Geometry check sheet. Reference: the model listing, model coordinates, mm. A direction names the side the tool comes from. Round coordinates to 2 decimals unless told otherwise and drop trailing zeros. Loops run counter-clockwise (first coordinate to the right, second up) from the corner with the lowest first, then second, coordinate; pieces in that order, holes last. Notation, with made-up numbers: M 49,50 L 94,50 A23 ccw 94,66 Z; hole C 9,-31.5 d9. An arc over 180 degrees is marked long. Write item = value, one per line.
from build123d import *

# Parameters (mm, degrees)
BOSS_EXTRUDE1_DEPTH     = 50.8
CUT_EXTRUDE1_DEPTH      = 26.4
CUT_EXTRUDE1_DEPTH_BACK = 1


with BuildPart() as part:
    # Sketch1 → Boss-Extrude1 (new body, symmetric)
    with BuildSketch(Plane(origin=(0, 0, 0), x_dir=(0, 0, -1), z_dir=(1, 0, 0))):
        Polygon((0, 0), (0, 25.4), (3.175, 25.4), (3.175, 3.175), (25.4, 3.175), (25.4, 0), align=None)
    extrude(amount=BOSS_EXTRUDE1_DEPTH, both=True)

    # Sketch2 → Cut-Extrude1 (cut, two sides)
    with BuildSketch(Plane(origin=(0, 0, 0), x_dir=(1, 0, 0), z_dir=(0, 1, 0))) as cut_extrude1_sk:
        Polygon((-50.8, 0), (-25.4, 25.4), (-50.8, 25.4), align=None)
        Polygon((50.8, 0), (50.8, 25.4), (25.4, 25.4), align=None)
    extrude(amount=CUT_EXTRUDE1_DEPTH, mode=Mode.SUBTRACT)
    extrude(cut_extrude1_sk.sketch, amount=-CUT_EXTRUDE1_DEPTH_BACK, mode=Mode.SUBTRACT)


solid = part.part
(1) Sectioned sample at D-D on x = -39.5. Record the cut outline in (y, z) (3 decimals).
Result set:
outline = M 0,-11.3 L 3.175,-11.3 L 3.175,-3.175 L 25.4,-3.175 L 25.4,0 L 0,0 Z
(2) Sectioned sample at B-B on z = -5.25. Record the cut outline in (x, y) (3 decimals).
Result set:
outline = M -45.55,0 L 45.55,0 L 45.55,3.175 L -45.55,3.175 Z
(3) Tool access check on faces 1 (the flat face through (1, 3.175, -14)), 2 (the flat face through (0, 2, -25.4)). Record the directions out of +Z, -Z, +X, -X, +Y, -Y that give a thin tool (end or side, any length) a straight path to the whole face; none if there is none.
Result set:
face_1 = -Z, +X, -X, +Y
face_2 = -Z, +X, -X, +Y, -Y
(4) Release check for a two-part mould opening along X. For faces 3 (the flat face through (1, 0, -10)), 4 (the flat face through (42.7, 2.3, -8.1)), 5 (the flat face through (-43.8, 2.3, -7)) record: released by +X, released by -X, zero draft, split by the parting line, or undercut.
Result set:
face_3 = zero draft
face_4 = released by +X
face_5 = released by -X
(5) Sectioned sample at C-C on y = 11.5. Record the cut outline in (x, z) (3 decimals).
Result set:
outline = M -50.8,0 L -47.625,-3.175 L 47.625,-3.175 L 50.8,0 Z
(6) Material ranges on line 1 along Z through (x, y) = (33, 3.5) (3 decimals); line 2 along Y through (x, z) = (-9, -18.75) (3 decimals); line 3 along Z through (x, y) = (-41, 2.5), recorded low to high. Write a range as from..to.
Result set:
line_1 = -3.175..0
line_2 = 0..3.175
line_3 = -9.8..0
(7) Sectioned sample at A-A on x = 28. Record the cut outline in (y, z) (3 decimals), then the cut area to 3 significant figures.
Result set:
outline = M 0,-22.8 L 3.175,-22.8 L 3.175,-3.175 L 25.4,-3.175 L 25.4,0 L 0,0 Z
area = 143 mm2
(8) Depth check by flat-ended pin: pin 1 Ø12 at (y, z) = (19.5, -12) entering from -X; pin 2 Ø6.5 at (x, z) = (-12.5, -12.5) entering from +Y (3 decimals); pin 3 Ø3 at (y, z) = (3, -8.5) entering from +X; pin 4 Ø2 at (y, z) = (3.5, -17) entering from +X. Enter the tip coordinate at first touch or a pass-through.
Result set:
pin_1 = through
pin_2 = 3.175
pin_3 = 43.8
pin_4 = 34.75
